```python
from build123d import *

# Parameters (mm, degrees)
CROQUIS1_R                          = 3
SALIENTE_EXTRUIR1_DEPTH             = 20
SALIENTE_EXTRUIR1_2_DEPTH           = 20
CROQUIS2_W                          = 142
CROQUIS2_H                          = 7
SALIENTE_EXTRUIR2_DEPTH             = 30
CROQUIS3_R                          = 27.5
SALIENTE_EXTRUIR3_DEPTH             = 70
SALIENTE_EXTRUIR3_DIRECTION_2_REACH = 89.121
CROQUIS4_R                          = 25
CORTAR_EXTRUIR1_DEPTH               = 70
CROQUIS5_R                          = 1
CORTAR_EXTRUIR2_DEPTH               = 5
CROQUIS6_R                          = 2.25
CORTAR_EXTRUIR3_DEPTH               = 10
REDONDEO1_R                         = 10
CORTAR_EXTRUIR4_DEPTH               = 117.052789712
CROQUIS8_R                          = 2
SALIENTE_EXTRUIR4_DEPTH             = 5
REDONDEO3_R                         = 5
CHAFL_N2_SIZE                       = 5
CHAFL_N1_SIZE                       = 2
CROQUIS9_R                          = 1.5
CORTAR_EXTRUIR5_DEPTH               = 109.019674134
CORTAR_EXTRUIR6_START               = -1
CROQUIS10_R                         = 25
CROQUIS10_R_2                       = 20
CORTAR_EXTRUIR6_DEPTH               = 1


with BuildPart() as part:
    # Croquis1 → Saliente-Extruir1 (new body)
    with BuildSketch(Plane(origin=(0, 0, 0), x_dir=(0, 0, -1), z_dir=(1, 0, 0))):
        with Locations((-65, 0)):
            Circle(CROQUIS1_R)
    extrude(amount=SALIENTE_EXTRUIR1_DEPTH)



with BuildPart() as body_2:
    # Croquis1 → Saliente-Extruir1 2 (new body)
    with BuildSketch(Plane(origin=(0, 0, 0), x_dir=(0, 0, -1), z_dir=(1, 0, 0))):
        with Locations((65, 0)):
            Circle(CROQUIS1_R)
    extrude(amount=SALIENTE_EXTRUIR1_2_DEPTH)


with BuildPart() as part_1:
    add(part.part)

    add(body_2.part)  # Saliente-Extruir2 merges body 2
    # Croquis2 → Saliente-Extruir2 (add)
    with BuildSketch(Plane(origin=(20, 0, 0), x_dir=(0, 0, -1), z_dir=(1, 0, 0))):
        Rectangle(CROQUIS2_W, CROQUIS2_H)
    extrude(amount=SALIENTE_EXTRUIR2_DEPTH)

    # Croquis3 → Saliente-Extruir3 (add)
    with BuildSketch(Plane.XZ.offset(3.5)):
        with Locations(Location((47.5, 0, 0), (0, 0, 270))):
            Circle(CROQUIS3_R)
    extrude(amount=SALIENTE_EXTRUIR3_DEPTH)

    # Saliente-Extruir3 direction 2: up to this face of the body (flat: up to its plane)
    saliente_extruir3_direction_2_end = Plane(part_1.part.faces().sort_by_distance((35, 3.5, 0))[0])
    # Croquis3 → Saliente-Extruir3 direction 2 (add, up to the picked face)
    with BuildSketch(Plane.XZ.offset(3.5), mode=Mode.PRIVATE) as saliente_extruir3_direction_2_sk1:
        with Locations(Location((47.5, 0, 0), (0, 0, 270))):
            Circle(CROQUIS3_R)
    saliente_extruir3_direction_2_tool1 = split(extrude(saliente_extruir3_direction_2_sk1.sketch, amount=-SALIENTE_EXTRUIR3_DIRECTION_2_REACH, mode=Mode.PRIVATE), bisect_by=saliente_extruir3_direction_2_end, keep=Keep.BOTH, mode=Mode.PRIVATE)
    add(saliente_extruir3_direction_2_tool1.solids().sort_by(Axis((47.5, -3.5, 0), (0, 1, 0)))[0])

    # Croquis4 → Cortar-Extruir1 (cut)
    with BuildSketch(Plane.XZ.offset(73.5)):
        with Locations(Location((47.5, 0, 0), (0, 0, 270))):
            Circle(CROQUIS4_R)
    extrude(amount=-CORTAR_EXTRUIR1_DEPTH, mode=Mode.SUBTRACT)

    # Croquis5 → Cortar-Extruir2 (cut)
    with BuildSketch(Plane.ZY):
        with Locations((-65, 0)):
            Circle(CROQUIS5_R)
        with Locations((65, 0)):
            Circle(CROQUIS5_R)
    extrude(amount=-CORTAR_EXTRUIR2_DEPTH, mode=Mode.SUBTRACT)

    # Croquis6 → Cortar-Extruir3 (cut)
    with BuildSketch(Plane(origin=(0, 3.5, 0), x_dir=(1, 0, 0), z_dir=(0, 1, 0))):
        with Locations(Location((35, 66, 0), (0, 0, 270))):
            Circle(CROQUIS6_R)
        with Locations(Location((35, 56, 0), (0, 0, 270))):
            Circle(CROQUIS6_R)
        with Locations(Location((35, -66, 0), (0, 0, 270))):
            Circle(CROQUIS6_R)
        with Locations(Location((35, -56, 0), (0, 0, 270))):
            Circle(CROQUIS6_R)
    extrude(amount=-CORTAR_EXTRUIR3_DEPTH, mode=Mode.SUBTRACT)

    # Redondeo1
    redondeo1_edges = [part_1.edges().sort_by_distance(p)[0] for p in [
        (50, 0, 71),
        (50, 0, -71),
    ]]
    fillet(redondeo1_edges, radius=REDONDEO1_R)

    # Croquis7 → Cortar-Extruir4 (cut, through all)
    with BuildSketch(Plane.ZY.offset(-20)):
        Polygon((-71, -3.5), (0, -3.5), (71, -3.5), (71, 3.5), (-71, 3.5), align=None)
    extrude(amount=CORTAR_EXTRUIR4_DEPTH, mode=Mode.SUBTRACT)

    # Croquis8 → Saliente-Extruir4 (add)
    # profile 1 of 2: a face of its own
    with BuildSketch(Plane.ZY.offset(-20)):
        with BuildLine():
            Line((-71, 10), (-71, -3.5))
            Line((-71, -3.5), (-59, -3.5))
            Line((-59, -3.5), (-59, 10))
            ThreePointArc((-59, 10), (-65, 16), (-71, 10))
        make_face()
        with Locations((-65, 10)):
            Circle(CROQUIS8_R, mode=Mode.SUBTRACT)
    # profile 2 of 2: a face of its own
    with BuildSketch(Plane.ZY.offset(-20)):
        with BuildLine():
            Line((59, 10), (59, -3.5))
            Line((59, -3.5), (71, -3.5))
            Line((71, -3.5), (71, 10))
            ThreePointArc((71, 10), (65, 16), (59, 10))
        make_face()
        with Locations(Location((65, 10, 0), (0, 0, 180))):
            Circle(CROQUIS8_R, mode=Mode.SUBTRACT)
    extrude(amount=SALIENTE_EXTRUIR4_DEPTH)

    # Redondeo3
    # the kernel refuses this fillet: 5 mm, written as the material it adds along each edge
    with BuildSketch(Plane(origin=(50, 3.5, -27.386127875), x_dir=(0, 0, -1), z_dir=(0, -1, 0))) as redondeo3_piece_1:
        with BuildLine():
            CenterArc((4.236648726, 5), REDONDEO3_R, 193.342363797, 76.657636203)
            ThreePointArc((-0.628393828, 3.846153846), (-0.245979187, 1.934222499), (0, 0))
            Line((0, 0), (4.236648726, 0))
        make_face()
    extrude(amount=7)
    with BuildSketch(Plane(origin=(50, 3.5, 27.386127875), x_dir=(0.9869144977622896, 0, -0.16124445449877534), z_dir=(0, -1, 0))) as redondeo3_piece_2:
        with BuildLine():
            CenterArc((4.251436376, 4.987432323), REDONDEO3_R, 189.279136184, 76.657636203)
            Line((-0.683136113, 4.18121005), (0, 0))
            ThreePointArc((0, 0), (1.948575006, 0.069122226), (3.897150011, 0))
        make_face()
    extrude(amount=7)
    # the kernel refuses this fillet: 5 mm, written as the material it takes off along each edge
    with BuildSketch(Plane(origin=(47.5, -73.5, 0), x_dir=(0, 0, -1), z_dir=(-1, 0, 0))) as redondeo3_2_piece_1:
        with BuildLine():
            CenterArc((22.5, -4.330127019), REDONDEO3_R, 0, 60)
            Line((25, 0), (27.5, 0))
            Line((27.5, 0), (27.5, -4.330127019))
        make_face()
    revolve(axis=Axis((47.5, -73.5, 0), (0, -1, 0)), mode=Mode.SUBTRACT)

    # Chaflán2
    # the kernel refuses this chamfer: 5 mm, written as the material it adds along each edge
    with BuildSketch(Plane(origin=(20, 3.5, 59), x_dir=(0, 0, -1), z_dir=(0, -1, 0)), Plane(origin=(20, -3.5, -59), x_dir=(0, 0, 1), z_dir=(0, 1, 0))) as chafl_n2_piece_1:
        Polygon((CHAFL_N2_SIZE, 0), (0, -CHAFL_N2_SIZE), (0, 0), align=None)
    extrude(amount=7)

    # Chaflán1
    chafl_n1_edges = [part_1.edges().sort_by_distance(p)[0] for p in [
        (20, 3.5, 65),
        (20, 3.5, -65),
    ]]
    chamfer(chafl_n1_edges, length=CHAFL_N1_SIZE)

    # Croquis9 → Cortar-Extruir5 (cut, through all)
    with BuildSketch(Plane(origin=(50, 0, 0), x_dir=(0, 0, -1), z_dir=(1, 0, 0))):
        with Locations(Location((0, -53.5, 0), (0, 0, 180))):
            Circle(CROQUIS9_R)
        with Locations(Location((0, -43.5, 0), (0, 0, 180))):
            Circle(CROQUIS9_R)
    extrude(amount=CORTAR_EXTRUIR5_DEPTH, mode=Mode.SUBTRACT)

    # Croquis10 → Cortar-Extruir6 (cut)
    with BuildSketch(Plane(origin=(0, 3.5, 0), x_dir=(1, 0, 0), z_dir=(0, 1, 0)).offset(CORTAR_EXTRUIR6_START)):
        with Locations(Location((47.5, 0, 0), (0, 0, 90))):
            Circle(CROQUIS10_R)
        with Locations(Location((47.5, 0, 0), (0, 0, 270))):
            Circle(CROQUIS10_R_2, mode=Mode.SUBTRACT)
    extrude(amount=CORTAR_EXTRUIR6_DEPTH, mode=Mode.SUBTRACT)


solid = part_1.part
```
Could you check a few things on this model? Use its own coordinates, in mm. A direction names the side the tool comes from. Round coordinates to 2 decimals unless told otherwise and drop trailing zeros. Write each loop counter-clockwise with the first axis right and the second up, starting at its lowest first coordinate (ties: lowest second). Pieces come first, ordered by that corner, then holes. Notation, with made-up numbers: M 85,62 L 138,62 A33 cw 138,91 Z; hole C 49.5,15.25 d4. An arc over 180 degrees is marked long. Write each question's results on one line, items separated by ' | '. Start each with the question number.
1. Imagine slicing it at C-C on z = -48. List the corners of the cut face in (x, y) for me, and give its area (3 significant figures).
2. Imagine slicing it at A-A on z = 56. List the corners of the cut face in (x, y) for me, and give its area (4 significant figures).
3. Imagine slicing it at D-D on x = 47.5. List the corners of the cut face in (y, z) for me, and give its area (3 significant figures).
4. I need wall thicknesses on L1, parallel to Z at x = 48, y = -57 (3 decimals); L2, parallel to Y at x = 73, z = 0; L3, parallel to Y at x = 19, z = -65. Which ranges of each line are inside material? Lowest first, please. Write a range as from..to.
5. Thinking about a two-plate mould opening in Z: for faces 6 (the face through (20, 12, 64)), 7 (the face through (36.52, 0.05, 64.34)), 8 (the face through (51.05, 0.05, 28.56)), which applies, +Z half, -Z half, draft (parallel to the pull), parting line (faces both ways), or undercut?
6. Imagine slicing it at B-B on y = -36. List the corners of the cut face in (x, z) for me.
7. I'm going to push flat-ended pins straight in: pin 1 Ø1.5 at (x, y) = (30.5, -63) entering from +Z; pin 2 Ø2 at (y, z) = (-61, 20) entering from +X; pin 3 Ø6 at (x, z) = (54.5, 11.5) entering from -Y. Where does each tip first touch, or does it pass through?
8. On a 3-axis mill with a long thin cutter (end or side, diameter ignored), from which of +Z, -Z, +X, -X, +Y, -Y can I reach the whole of each face in a straight line? I mean faces 1 (the face through (23.094, -38.99, 5.42)), 2 (the face through (50, 0, -46)), 3 (the face through (20, 12, -66)), 4 (the face through (74, -42, 0)), 5 (the face through (67.33, 2.99, -2.6)). Say none if no direction works.
Result sheet:
1) outline: M 20,-3.5 L 50,-3.5 L 50,3.5 L 20,3.5 Z | area: 210 mm^2
2) outline: M 18,-3.5 L 32.75,-3.5 L 32.75,3.5 L 18,3.5 Z; M 37.25,-3.5 L 50,-3.5 L 50,3.5 L 37.25,3.5 Z | area: 192.5 mm^2
3) outline: M -73.5,-25 A5 ccw -69.17,-27.5 L -3.5,-27.5 L -3.5,-67.61 L 3.5,-67.61 L 3.5,-25 L 2.5,-25 L 2.5,-20 L 3.5,-20 L 3.5,20 L 2.5,20 L 2.5,25 L 3.5,25 L 3.5,67.61 L -3.5,67.61 L -3.5,27.5 L -69.17,27.5 A5 ccw -73.5,25 L -3.5,25 L -3.5,-25 Z | area: 1,280 mm^2
4) L1: z = -27.495..-24.995, 24.995..27.495 | L2: y = -73.17..-55, -52..-45, -42..3.5 | L3: y = -3.5..8, 12..16
5) face 6: draft | face 7: undercut | face 8: +Z half
6) outline: C 47.5,0 d55; hole C 47.5,0 d50
7) pin 1: stops at z = 22.19 | pin 2: stops at x = 67.38 | pin 3: stops at y = -3.5
8) face 1: -Y | face 2: -Z, +X, +Y, -Y | face 3: +Z, -Z, +X, +Y | face 4: +X | face 5: +Y
